Autodesk Inventor part; units mm, degrees
ref_plane "YZ Plane" through (0, 0, 0) normal (1, 0, 0) x (0, 1, 0)
ref_plane "XZ Plane" through (0, 0, 0) normal (0, 1, 0) x (-1, 0, 0)
ref_plane "XY Plane" through (0, 0, 0) normal (0, 0, 1) x (1, 0, 0)
sketch "Sketch1" plane through (0, 0, 0) normal (0, 1, 0) x (-1, 0, 0)
  circle A0 centre (0, 0) radius 3.5
  circle A1 centre (0, 0) radius 6
  line L0 (0, 0) -> (0, -20)
  line L1 (25, -20) -> (-25, -20)
  line L2 (25, -20) -> (4.5598, 3.8998)
  line L3 (-25, -20) -> (-4.5598, 3.8998)
  line L4 (25, -20) -> (-25, -20)
  line L5 (-25, -20) -> (-25, -23)
  line L6 (-25, -23) -> (25, -23)
  line L7 (25, -23) -> (25, -20)
  point P0 (-25, -20)
  dimension "d0" = 7
  dimension "d1" = 12
  dimension "d2" = 20
  dimension "d3" = 50
  dimension "d4" = 3
extrude "Extrusion1" add sketch "Sketch1" along normal blind 21
sketch "Sketch2" plane through (0, 0, 0) normal (1, 0, 0) x (0, 1, 0)
  line L0 (18, -20) -> (3, -20)
  line L1 (3, -20) -> (3, 27.9628)
  line L2 (3, 27.9628) -> (18, 27.9628)
  line L3 (18, 27.9628) -> (18, -20)
  line L4 (0, -20) -> (21, -20)
  point P0 (0, 0)
  point P1 (10.5, -20)
  dimension "d7" = 15
extrude "Extrusion2" cut sketch "Sketch2" along normal mid plane 100
properties part number "ShifterBracket"
Design review of the part built by this model. Coordinates are the model's own, in mm. A direction names the side the tool comes from. Round coordinates to 2 decimals unless told otherwise and drop trailing zeros. Write each loop counter-clockwise with the first axis right and the second up, starting at its lowest first coordinate (ties: lowest second). Pieces come first, ordered by that corner, then holes.
Item 1: Consider section A-A on x = 0. Give the boundary of the cut face in (y, z).
Item 2: Wall thickness on L1, parallel to Y at x = -3, z = 3.75; L2, parallel to Z at x = -12.5, y = 17.25; L3, parallel to X at y = 19.5, z = -2.25: over which ranges is each line inside the solid? List them lowest first.
Item 3: Consider section B-B on z = 1.25. Give the boundary of the cut face in (x, y).
Item 4: Draft analysis for pull direction X (two halves, no side actions). For faces 3 (the flat face through (0, 11, -20)), 4 (the cylindrical face through (-3.233, 19.479, 1.341)), 5 (the flat face through (-14.923, 19.479, -8.217)), 6 (the cylindrical face through (-3.233, 1.479, 1.341)), state which applies: released by +X, released by -X, zero draft, split by the parting line, or undercut.
Item 5: Consider section C-C on z = -9.75. Give the boundary of the cut face in (x, y).
Item 6: For faces 1 (the flat face through (-14.923, 1.479, -8.217)), 2 (the flat face through (0, 3, -10)), list the 3-axis set-ups (+Z, -Z, +X, -X, +Y, -Y) from which the entire face can be reached by the end or side of a thin tool; tool diameter is ignored.
Item 7: Consider section D-D on x = -16. Give the boundary of the cut face in (y, z), and give its area (3 significant figures).
Item 8: For pin 1 Ø10 at (x, z) = (16, -10) entering from -Y; pin 2 Ø5 at (y, z) = (2, -15.5) entering from +X; pin 3 Ø4 at (x, y) = (1, 15.5) entering from +Z, all flat-tipped, find the tip position at first contact; note any pin that passes through.
Check values:
1. outline: (0, -23) - (21, -23) - (21, -3.5) - (18, -3.5) - (18, -20) - (3, -20) - (3, -3.5) - (0, -3.5) - close; (0, 3.5) - (3, 3.5) - (3, 6) - (0, 6) - close; (18, 3.5) - (21, 3.5) - (21, 6) - (18, 6) - close
2. L1: y = 0 to 3, 18 to 21
2. L2: z = -23 to -20
2. L3: x = -9.82 to -2.68, 2.68 to 9.82
3. outline: (-6.83, 0) - (-3.27, 0) - (-3.27, 3) - (-6.83, 3) - close; (-6.83, 18) - (-3.27, 18) - (-3.27, 21) - (-6.83, 21) - close; (3.27, 0) - (6.83, 0) - (6.83, 3) - (3.27, 3) - close; (3.27, 18) - (6.83, 18) - (6.83, 21) - (3.27, 21) - close
4. face 3: zero draft
4. face 4: undercut
4. face 5: released by -X
4. face 6: undercut
5. outline: (-16.23, 0) - (16.23, 0) - (16.23, 3) - (-16.23, 3) - close; (-16.23, 18) - (16.23, 18) - (16.23, 21) - (-16.23, 21) - close
6. face 1: +Z, -X, +Y, -Y
6. face 2: +Z, +X, -X
7. outline: (0, -23) - (21, -23) - (21, -9.48) - (18, -9.48) - (18, -20) - (3, -20) - (3, -9.48) - (0, -9.48) - close
7. area: 126 mm2
8. pin 1: stops at y = 0
8. pin 2: stops at x = 23.29
8. pin 3: stops at z = -20
